The listing builds one solid part. Answer for the finished solid, in the listing's coordinates (mm). A direction names the side the tool comes from. Round coordinates to 2 decimals unless told otherwise and drop trailing zeros. Loops run counter-clockwise (first coordinate to the right, second up) from the corner with the lowest first, then second, coordinate; pieces in that order, holes last. Notation, with made-up numbers: (15, 35) -> (52, 35) arc R20 ccw to (52, 74) -> close; hole circle Ø9 at (5, -36). An arc over 180 degrees is marked (long way). Answer in a Markdown table with one row per item. Add a question column.
```python
from build123d import *

# Parameters (mm, degrees)
BOSS_EXTRUDE4_DEPTH = 20
CUT_EXTRUDE1_DEPTH  = 89.134124702


with BuildPart() as part:
    # Sketch1 → Boss-Extrude4 (new body)
    with BuildSketch(Plane.XY):
        Polygon((-32.575757576, -52.904040404), (-36.334940312, 46.338383838), (22.727272727, 46.338383838), (47.853859566, 12.836268054), (22.727272727, -5.850467639), (67.592798773, -39.94137673), (57.74316526, -52.904040404), align=None)
    extrude(amount=BOSS_EXTRUDE4_DEPTH)

    # Sketch3 → Cut-Extrude1 (cut, through all)
    with BuildSketch(Plane.XY.offset(20)):
        Polygon((10.494111386, -9.114469372), (-5.575689301, -9.114469372), (-14.041829745, 2.173717887), (16.759656232, 2.173717887), (33.829559486, 14.868668159), (17.727272727, 36.338383838), (-25.948980992, 36.338383838), (-22.947374013, -42.904040404), (52.782303891, -42.904040404), (53.580530259, -41.853530257), align=None)
    extrude(amount=-CUT_EXTRUDE1_DEPTH, mode=Mode.SUBTRACT)


solid = part.part
```
Item 1: Section A-A, the plane x = 3 is taken. Write down the section's boundary in (y, z), and give its area (3 significant figures).
Item 2: The mould has two halves that part along X. Classify faces 4 (the flat face through (-24.47, -2.73, 10.14)), 5 (the flat face through (-7, 46.338, 10)), 6 (the flat face through (-34.43, -3.98, 9.86)), 7 (the flat face through (62.74, -46.33, 9.86)): +X half, -X half, draft (parallel to the pull), parting line (faces both ways), or undercut.
Item 3: Section D-D, the plane y = -7.5 is taken. Write down the section's boundary in (x, z).
Item 4: Section C-C, the plane x = -19 is taken. Write down the section's boundary in (y, z), and give its area (3 significant figures).
Item 5: Consider L1, parallel to Y at x = 6.5, z = 1.5; L2, parallel to Y at x = 25, z = 9; L3, parallel to Y at x = 36, z = 18. Determine where each line is inside the solid, lowest interval first. Write a range as from..to.
Item 6: For faces 1 (the flat face through (44.85, -22.66, 9.86)), 2 (the flat face through (5, -3, 20)), 3 (the flat face through (25.175, 8.432, 10.14)), determine the directions among +Z, -Z, +X, -X, +Y, -Y from which every point of the face is accessible in a straight line to the end or side of a thin tool.
Item 7: Flat-ended cylindrical pins translate along their axes: P1, Ø10, axis at y = -25.5, z = 9.5, coming from the -X side; P2, Ø1.5, axis at x = 31.5, y = 5, coming from the -Z side; P3, Ø5, axis at y = -19, z = 15.5, coming from the +X side. Find the tip coordinate at first contact, or state that the pin passes through.
Item 8: Section B-B, the plane z = 16.5 is taken. Write down the section's boundary in (x, y), and give its area (3 significant figures).
Here are the results:
| question | item | result |
|---|---|---|
| 1 | outline | (-52.9, 0) -> (-42.9, 0) -> (-42.9, 20) -> (-52.9, 20) -> close; (-9.11, 0) -> (2.17, 0) -> (2.17, 20) -> (-9.11, 20) -> close; (36.34, 0) -> (46.34, 0) -> (46.34, 20) -> (36.34, 20) -> close |
| 1 | area | 626 mm² |
| 2 | face 4 | undercut |
| 2 | face 5 | draft |
| 2 | face 6 | -X half |
| 2 | face 7 | +X half |
| 3 | outline | (-34.3, 0) -> (-24.29, 0) -> (-24.29, 20) -> (-34.3, 20) -> close; (-6.79, 0) -> (24.9, 0) -> (24.9, 20) -> (-6.79, 20) -> close |
| 4 | outline | (-52.9, 0) -> (-42.9, 0) -> (-42.9, 20) -> (-52.9, 20) -> close; (36.34, 0) -> (46.34, 0) -> (46.34, 20) -> (36.34, 20) -> close |
| 4 | area | 400 mm² |
| 5 | L1 | y = -52.9..-42.9, -9.11..2.17, 36.34..46.34 |
| 5 | L2 | y = -52.9..-42.9, -20.14..-7.58, -4.16..8.3, 26.64..43.31 |
| 5 | L3 | y = -52.9..-42.9, -28.5..-15.94, 4.02..28.64 |
| 6 | face 1 | +Z, -Z, +X |
| 6 | face 2 | +Z, +X, -X, +Y, -Y |
| 6 | face 3 | +Z, -Z |
| 7 | P1 | stops at x = -33.8 |
| 7 | P2 | stops at z = 0 |
| 7 | P3 | stops at x = 43.32 |
| 8 | outline | (-36.33, 46.34) -> (-32.58, -52.9) -> (57.74, -52.9) -> (67.59, -39.94) -> (22.73, -5.85) -> (47.85, 12.84) -> (22.73, 46.34) -> close; hole (-25.95, 36.34) -> (-22.95, -42.9) -> (52.78, -42.9) -> (53.58, -41.85) -> (10.49, -9.11) -> (-5.58, -9.11) -> (-14.04, 2.17) -> (16.76, 2.17) -> (33.83, 14.87) -> (17.73, 36.34) -> close |
| 8 | area | 3,810 mm² |
